from build123d import *

# Parameters (mm, degrees)
SKETCH1_W           = 40
SKETCH1_H           = 50
BOSS_EXTRUDE1_DEPTH = 25
SKETCH2_R           = 8
CUT_EXTRUDE1_DEPTH  = 58
SKETCH3_R           = 3
CUT_EXTRUDE2_DEPTH  = 25


with BuildPart() as part:
    # Sketch1 → Boss-Extrude1 (new body)
    with BuildSketch(Plane.XY):
        with Locations((20, 25)):
            Rectangle(SKETCH1_W, SKETCH1_H)
    extrude(amount=BOSS_EXTRUDE1_DEPTH)

    # Sketch2 → Cut-Extrude1 (cut)
    with BuildSketch(Plane.ZY):
        with Locations((25, 25)):
            Circle(SKETCH2_R)
    extrude(amount=-CUT_EXTRUDE1_DEPTH, mode=Mode.SUBTRACT)

    # Sketch3 → Cut-Extrude2 (cut)
    with BuildSketch(Plane.XY.offset(25)):
        with Locations((10, 40)):
            Circle(SKETCH3_R)
        with Locations((30, 40)):
            Circle(SKETCH3_R)
        with Locations((30, 10)):
            Circle(SKETCH3_R)
        with Locations((10, 10)):
            Circle(SKETCH3_R)
    extrude(amount=-CUT_EXTRUDE2_DEPTH, mode=Mode.SUBTRACT)


solid = part.part
Source: CAD feature listing. Evaluate the final solid. Frame: model axes, mm. Coordinates: 2 decimals unless noted, no trailing zeros. Loops run counter-clockwise (first coordinate to the right, second up) from the corner with the lowest first, then second, coordinate; pieces in that order, holes last. Notation, with made-up numbers: (36, 25.5) - (90, 25.5) arc R19 cw to (90, 38.5) - close; hole circle Ø4 at (77.25, 69). An arc over 180 degrees is marked (long way). Return JSON: item names as keys, results as strings.
Q1. Contact query for a flat-ended pin moving along its axis: P1, Ø5.5, axis at x = 10, y = 10, coming from the +Z side. Output: stop coordinate, or through.
Results:
{"P1": "through"}
Q2. Mould query, pull axis Y, two halves, no side actions, for faces 1 (the cylindrical face through (27, 10, 13)), 2 (the flat face through (20, 50, 12)), 3 (the flat face through (0, 25, 12)), 4 (the cylindrical face through (20, 25, 17)). Classes: released by +Y, released by -Y, zero draft, split by the parting line, or undercut.
Results:
{"face 1": "undercut", "face 2": "released by +Y", "face 3": "zero draft", "face 4": "undercut"}
Q3. Section B-B, the plane y = 40. Return loops of the section in (x, z), plus the area to 3 significant figures.
Results:
{"outline": "(0, 0) - (7, 0) - (7, 25) - (0, 25) - close; (13, 0) - (27, 0) - (27, 25) - (13, 25) - close; (33, 0) - (40, 0) - (40, 25) - (33, 25) - close", "area": "700 mm2"}
Q4. Section D-D, the plane z = 9.5. Return loops of the section in (x, y), plus the area to 3 significant figures.
Results:
{"outline": "(0, 0) - (40, 0) - (40, 50) - (0, 50) - close; hole circle Ø6 at (10, 10); hole circle Ø6 at (10, 40); hole circle Ø6 at (30, 10); hole circle Ø6 at (30, 40)", "area": "1,890 mm2"}
Q5. Material intervals for line 1 along Y through (x, z) = (30, 9.5); line 2 along Y through (x, z) = (8.5, 14); line 3 along Y through (x, z) = (31, 21), sorted ascending.
Results:
{"line 1": "0 to 7, 13 to 37, 43 to 50", "line 2": "0 to 7.4, 12.6 to 37.4, 42.6 to 50", "line 3": "0 to 7.17, 12.83 to 18.07, 31.93 to 37.17, 42.83 to 50"}
Q6. Section A-A, the plane x = 30. Return loops of the section in (y, z), plus the area to 3 significant figures.
Results:
{"outline": "(0, 0) - (7, 0) - (7, 25) - (0, 25) - close; (13, 0) - (37, 0) - (37, 25) - (33, 25) arc R8 cw to (17, 25) - (13, 25) - close; (43, 0) - (50, 0) - (50, 25) - (43, 25) - close", "area": "849 mm2"}
Q7. Section C-C, the plane z = 22.75. Return loops of the section in (x, y), plus the area to 3 significant figures.
Results:
{"outline": "(0, 0) - (40, 0) - (40, 17.32) - (0, 17.32) - close; (0, 32.68) - (40, 32.68) - (40, 50) - (0, 50) - close; hole circle Ø6 at (10, 10); hole circle Ø6 at (10, 40); hole circle Ø6 at (30, 10); hole circle Ø6 at (30, 40)", "area": "1,270 mm2"}
